from build123d import *

# Parameters (mm, degrees)
F0_R     = 3.5
F1_DEPTH = 10
F2_R     = 0.5
F3_R     = 0.5
F4_DEPTH = 3.5


with BuildPart() as f1:
    # F0 (on Front) → F1 (new body)
    with BuildSketch(Plane.XZ):
        Circle(F0_R)
    extrude(amount=F1_DEPTH)

    # F2
    f2_edges = [f1.edges().sort_by_distance(p)[0] for p in [
        (-3.5, -10, 0),
    ]]
    fillet(f2_edges, radius=F2_R)

    # F3 (on face) → F4 (join)
    with BuildSketch(Plane.XZ.offset(10)):
        Circle(F3_R)
    extrude(amount=F4_DEPTH)


solid = f1.part
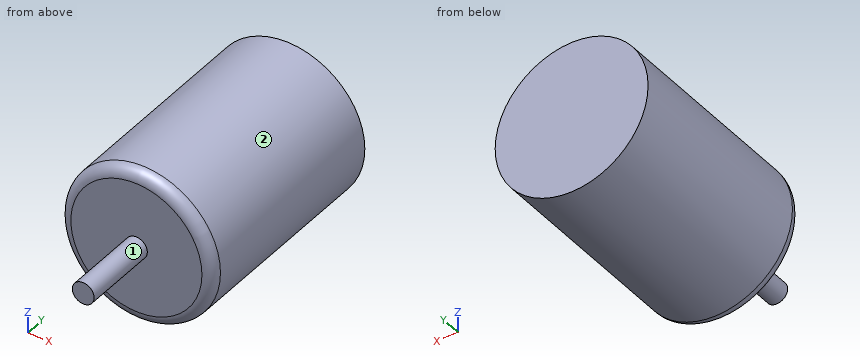
Verification items for the finished model (mm, model axes). Face numbers are marked on the shaded views. A direction names the side the tool comes from. Coordinates: 2 decimals unless noted, no trailing zeros. Write each loop counter-clockwise with the first axis right and the second up, starting at its lowest first coordinate (ties: lowest second). Pieces come first, ordered by that corner, then holes. Notation, with made-up numbers: (73, 47.5) - (99, 47.5) arc R21 cw to (99, 70.5) - close; hole circle Ø10 at (65, -27). An arc over 180 degrees is marked (long way). Answer as a JSON object with one key per item and string values.
(1) Cross-section at A-A on z = 0. Record the cut outline in (x, y).
Report:
{"outline": "(-3.5, -9.5) arc R0.5 ccw to (-3, -10) - (-0.5, -10) - (-0.5, -13.5) - (0.5, -13.5) - (0.5, -10) - (3, -10) arc R0.5 ccw to (3.5, -9.5) - (3.5, 0) - (-3.5, 0) - close"}
(2) Thickness scan on line 1 along Y through (x, z) = (-1, -1.5); line 2 along Z through (x, y) = (-1, -9.5); line 3 along Z through (x, y) = (2.5, -9.75). Record the ranges inside material, lowest first.
Report:
{"line 1": "-10 to 0", "line 2": "-3.35 to 3.35", "line 3": "-2.35 to 2.35"}
(3) Gauge pin test, flat ends, axial feed: pin 1 Ø3 at (y, z) = (-11, 0.5) entering from +X; pin 2 Ø1.5 at (x, y) = (1, -11.5) entering from +Z. Record the tip position at first contact, or that the pin passes through.
Report:
{"pin 1": "x = 3.5", "pin 2": "z = 0.43"}
(4) Tool access check on the marked faces 1 and 2. Record the directions out of +Z, -Z, +X, -X, +Y, -Y that give a thin tool (end or side, any length) a straight path to the whole face; none if there is none.
Report:
{"face 1": "-Y", "face 2": "+Y, -Y"}
(5) Cross-section at D-D on y = -9.75. Record the cut outline in (x, z).
Report:
{"outline": "circle Ø6.87 at (0, 0)"}
(6) Cross-section at B-B on x = 0. Record the cut outline in (y, z), plus the area to 3 significant figures.
Report:
{"outline": "(-13.5, -0.5) - (-10, -0.5) - (-10, -3) arc R0.5 ccw to (-9.5, -3.5) - (0, -3.5) - (0, 3.5) - (-9.5, 3.5) arc R0.5 ccw to (-10, 3) - (-10, 0.5) - (-13.5, 0.5) - close", "area": "73.4 mm^2"}
(7) Cross-section at C-C on y = -1.5. Record the cut outline in (x, z).
Report:
{"outline": "circle Ø7 at (0, 0)"}
